Could you check a few things on this model? Use its own coordinates, in mm. Face numbers are marked on the shaded views. A direction names the side the tool comes from. Give positions to 0.01 mm unless a question says otherwise; leave off trailing zeros. Loops run counter-clockwise (first coordinate to the right, second up) from the corner with the lowest first, then second, coordinate; pieces in that order, holes last. Notation, with made-up numbers: (29, -14) - (50, -14) arc R22 cw to (50, -4) - close; hole circle Ø3 at (85, -3). An arc over 180 degrees is marked (long way). Write each question's results on one line, items separated by ' | '. Start each with the question number.
(1) If we mould it in two halves opening along X, with no side actions, what happens to the marked faces 1, 2 and 3? For each: released by +X, released by -X, zero draft, split by the parting line, or undercut.
(2) I need wall thicknesses on line 1 (Y direction, x = -27.2, z = -25); line 2 (X direction, y = -11.75, z = -18.5); line 3 (Z direction, x = -84.5, y = -3.75). Which ranges of each line are inside material? Lowest first, please.
(3) Suppose I cut it at A-A (z = -13.5). Please give me the cut outline in (x, y), and give its area (3 significant figures).
(4) On a 3-axis mill with a long thin cutter (end or side, diameter ignored), from which of +Z, -Z, +X, -X, +Y, -Y can I reach the whole of each face in a straight line? I mean the marked faces 4, 5, 6, 7 and 8. Say none if no direction works.
(5) Suppose I cut it at C-C (z = -25). Please give me the cut outline in (x, y).
(6) For pin 1 (6 mm diameter, centred on y = -14.5, z = -8.5, fed in from -X); pin 2 (7.5 mm diameter, centred on x = -92.5, y = -11, fed in from +Z); pin 3 (8 mm diameter, centred on x = -91.99, y = -10, fed in from -Z), each with a flat end and sliding along its axis, tell me the tip position at first contact or that it passes through.
(7) Suppose I cut it at B-B (z = -8.5). Please give me the cut outline in (x, y).
(8) Suppose I cut it at D-D (y = -5.25). Please give me the cut outline in (x, z).
from build123d import *

# Parameters (mm, degrees)
SKETCH2_R           = 15
BOSS_EXTRUDE1_DEPTH = 20
SKETCH3_R           = 3.5
CUT_EXTRUDE1_DEPTH  = 36.5
SKETCH4_R           = 3.5
CUT_EXTRUDE2_DEPTH  = 36.5


with BuildPart() as part:
    # Sketch2 → Boss-Extrude1 (new body)
    with BuildSketch(Plane(origin=(0, 0, 0), x_dir=(1, 0, 0), z_dir=(0, 1, 0))):
        with BuildLine():
            Line((0, 0), (0, 30))
            Line((0, 30), (-5, 30))
            Line((-5, 30), (-5, 15))
            Line((-5, 15), (-25, 15))
            Line((-25, 15), (-25, 30))
            Line((-25, 30), (-30, 30))
            Line((-30, 30), (-30, 15))
            Line((-30, 15), (-45.987731213, 15))
            ThreePointArc((-45.987731213, 15), (-63.987731213, 26.282202113), (-81.987731213, 15))
            Line((-81.987731213, 15), (-96.987731213, 15))
            Line((-96.987731213, 15), (-96.987731213, 10))
            Line((-96.987731213, 10), (-83.639142838, 10))
            ThreePointArc((-83.639142838, 10), (-83.950029119, 7.509663844), (-83.946587837, 5))
            Line((-83.946587837, 5), (-97.975462426, 5))
            Line((-97.975462426, 5), (-97.975462426, 0))
            Line((-97.975462426, 0), (-82.975462426, 0))
            ThreePointArc((-82.975462426, 0), (-63.987731213, -13.717797887), (-45, 0))
            Line((-45, 0), (0, 0))
        make_face()
        with Locations(Location((-63.987731213, 6.282202113, 0), (0, 0, 270))):
            Circle(SKETCH2_R, mode=Mode.SUBTRACT)
    extrude(amount=-BOSS_EXTRUDE1_DEPTH)

    # Sketch3 → Cut-Extrude1 (cut, symmetric)
    with BuildSketch(Plane(origin=(0, 0, 0), x_dir=(0, 0, -1), z_dir=(1, 0, 0))):
        with Locations((25, -10)):
            Circle(SKETCH3_R)
    extrude(amount=CUT_EXTRUDE1_DEPTH, both=True, mode=Mode.SUBTRACT)

    # Sketch4 → Cut-Extrude2 (cut, symmetric)
    with BuildSketch(Plane(origin=(0, 0, -15), x_dir=(-1, 0, 0), z_dir=(0, 0, -1))):
        with Locations((91.987731213, -10)):
            Circle(SKETCH4_R)
    extrude(amount=CUT_EXTRUDE2_DEPTH, both=True, mode=Mode.SUBTRACT)


solid = part.part
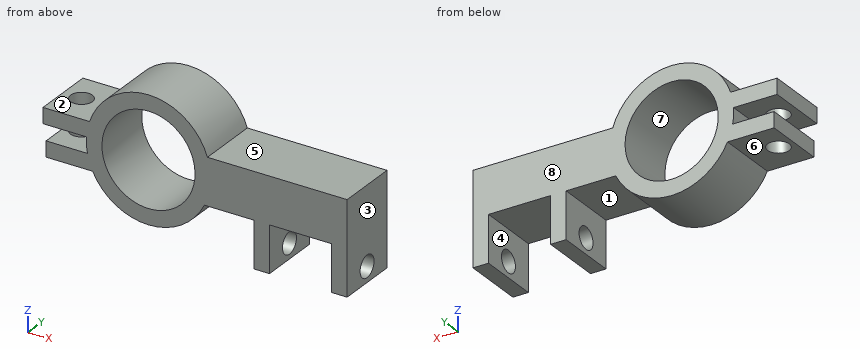
Output values:
1) face 1: undercut | face 2: zero draft | face 3: released by +X
2) line 1: -20 to -13.5, -6.5 to 0 | line 2: -79.82 to -72.69, -55.29 to -48.15, -30 to -25, -5 to 0 | line 3: -15 to -10, -5 to 0
3) outline: (-96.99, -20) - (-77.14, -20) - (-77.14, 0) - (-96.99, 0) - close; (-50.84, -20) - (0, -20) - (0, 0) - (-50.84, 0) - close; hole circle Ø7 at (-91.99, -10) | area: 1,380 mm2
4) face 4: -Z, +Y, -Y | face 5: +Z, +X, +Y, -Y | face 6: -Z, -X, +Y, -Y | face 7: +Y, -Y | face 8: +Z, -Z, +X, -X, +Y
5) outline: (-71.03, -20) - (-56.94, -20) - (-56.94, 0) - (-71.03, 0) - close; (-30, -20) - (-25, -20) - (-25, -13.5) - (-30, -13.5) - close; (-30, -6.5) - (-25, -6.5) - (-25, 0) - (-30, 0) - close; (-5, -20) - (0, -20) - (0, -13.5) - (-5, -13.5) - close; (-5, -6.5) - (0, -6.5) - (0, 0) - (-5, 0) - close
6) pin 1: x = -96.99 | pin 2: z = 0 | pin 3: z = -15
7) outline: (-83.86, -20) - (-78.82, -20) - (-78.82, 0) - (-83.86, 0) - close; (-49.15, -20) - (0, -20) - (0, 0) - (-49.15, 0) - close
8) outline: (-97.98, -5) - (-83.95, -5) arc R20 ccw to (-83.64, -10) - (-96.99, -10) - (-96.99, -15) - (-81.99, -15) arc R20 ccw to (-45.99, -15) - (-30, -15) - (-30, -30) - (-25, -30) - (-25, -15) - (-5, -15) - (-5, -30) - (0, -30) - (0, 0) - (-45, 0) arc R20 ccw to (-82.98, 0) - (-97.98, 0) - close; hole circle Ø30 at (-63.99, -6.28)
